Autodesk Inventor part; units mm, degrees
ref_plane "YZ Plane" through (0, 0, 0) normal (1, 0, 0) x (0, 1, 0)
ref_plane "XZ Plane" through (0, 0, 0) normal (0, 1, 0) x (-1, 0, 0)
ref_plane "XY Plane" through (0, 0, 0) normal (0, 0, 1) x (1, 0, 0)
sketch "Boceto1" plane through (0, 0, 0) normal (0, 1, 0) x (-1, 0, 0)
  line L0 (0, 0) -> (22, 0)
  line L1 (22, 0) -> (22, -15)
  line L2 (22, -15) -> (0, -15)
  line L3 (0, -15) -> (-12, -15)
  line L4 (-12, -15) -> (-12, 0)
  line L5 (-12, 0) -> (0, 0)
  dimension "d15" = 12
extrude "Extrusión1" add sketch "Boceto1" along normal blind 3
sketch "Boceto3" plane through (0, 3, 0) normal (0, 1, 0) x (1, 0, 0)
  line L0 (-22, 15) -> (-22, 0)
  line L1 (-22, 15) -> (-27, 15)
  line L2 (-27, 15) -> (-27, 0)
  line L3 (-27, 0) -> (-22, 0)
  line L4 (-22, 0) -> (-22, 15)
  point P0 (0, 0)
  dimension "d4" = 5
extrude "Extrusión2" add sketch "Boceto3" against normal blind 57
sketch "Boceto4" plane through (-22, -54, 0) normal (1, 0, 0) x (0, 0, -1)
  point P0 (0, 54)
sketch "Boceto5" plane through (-22, -54, 0) normal (1, 0, 0) x (0, 0, -1)
  line L0 (0, 57) -> (0, 0)
  line L1 (15, 57) -> (15, 0)
  line L2 (0, 0) -> (15, 0)
  line L3 (15, 0) -> (15, 3.0333)
  line L4 (15, 3.0333) -> (0, 3.0333)
  line L5 (0, 3.0333) -> (0, 0)
  point P0 (0, 54)
extrude "Extrusión3" add sketch "Boceto5" along normal blind 12
sketch "Boceto7" plane through (12, 0, 0) normal (1, 0, 0) x (0, 0, -1)
  line L0 (0, 0) -> (0, -50.9667)
  line L1 (0, 3) -> (0, 0)
  line L2 (0, 0) -> (0, -7)
  line L3 (0, -7) -> (10.8666, -7)
  line L4 (0, -7) -> (0, -13)
  line L5 (0, -13) -> (15, -13)
  line L6 (15, 0) -> (15, -50.9667)
  line L7 (15, 3) -> (15, -54)
  line L8 (15, 3) -> (15, -13)
  line L9 (15, 3) -> (0, 3)
  line L10 (15, 3) -> (0, 3)
  line L11 (0, 3) -> (0, -13)
  line L12 (0, -7) -> (15, -7)
  circle A0 centre (7.5, -7) radius 1.5
  dimension "d16" = 7
  dimension "d17" = 6
  dimension "d18" = 3
extrude "Extrusión5" add sketch "Boceto7" along normal blind 6 contours L1 L9 L7 L6 L12 L3 A0 L0 | L3 A0 L12 L6 L5 L0
sketch "Boceto8" plane through (-22, 0, 0) normal (1, 0, 0) x (0, 0, -1)
  line L0 (15, -50.9667) -> (0, -50.9667)
  line L1 (0, -50.9667) -> (0, -40.9667)
  line L2 (0, 0) -> (0, -50.9667)
  line L3 (0, -40.9667) -> (0, -38.9667)
  line L4 (0, -38.9667) -> (15, -38.9667)
  line L5 (15, 0) -> (15, -50.9667)
  line L6 (0, -40.9667) -> (15, -40.9667)
  line L7 (15, -40.9667) -> (15, -38.9667)
  dimension "d21" = 10
  dimension "d22" = 2
extrude "Extrusión6" add sketch "Boceto8" along normal blind 6 contours L6 L2 L4 L5
sketch "Boceto9" plane through (-22, -38.9667, 0) normal (0, 1, 0) x (1, 0, 0)
  line L0 (0, 0) -> (0, 15)
  line L1 (0, 0) -> (0, 15)
  line L2 (6, 15) -> (6, 0)
  line L3 (0, 15) -> (6, 15)
  line L4 (6, 15) -> (6, 0)
  line L5 (0, 15) -> (0, 0)
  line L6 (6, 0) -> (0, 0)
  point P0 (22, 0)
extrude "Extrusión7" add sketch "Boceto9" along normal blind 18
properties part number "agarre motor"
The model under review builds one solid part; all positions refer to its coordinate system, in mm. A direction names the side the tool comes from. Coordinates: 2 decimals unless noted, no trailing zeros. Loops run counter-clockwise (first coordinate to the right, second up) from the corner with the lowest first, then second, coordinate; pieces in that order, holes last. Notation, with made-up numbers: (4.5, 1) -> (42.5, 1) arc R19 cw to (42.5, 13) -> close; hole circle Ø5 at (21.25, 72.25). An arc over 180 degrees is marked (long way). Use a Markdown table: item, result. Add a question column.
1. Draft analysis for pull direction X (two halves, no side actions). For faces 1 (the face through (-27, -25, -8)), 2 (the face through (-5, 0, -7)), 3 (the face through (-19, -54, -7)), 4 (the face through (-10, -52, -7)), state which applies: pulls with the +X half, pulls with the -X half, needs draft (parallel to the pull), parting line crosses it, or undercut.
2. Add section B-B on y = -7. Write out the cut boundary in (x, z).
3. To check wall thickness, follow line 1 (Y direction, x = -20, z = -4); line 2 (Z direction, x = 15.6, y = -7); line 3 (Y direction, x = 16.2, z = -7.5). State the ranges of each line that lie inside material, in increasing order.
4. Add section A-A on x = -19.5. Write out the cut boundary in (y, z), plus the area to 4 significant figures.
5. Clearance check with flat-ended pins moving along their axes: pin 1 Ø3 at (y, z) = (-44, -6.5) entering from +X; pin 2 Ø1.5 at (y, z) = (-52, -5) entering from +X; pin 3 Ø12 at (x, y) = (5, -3.5) entering from -Z; pin 4 Ø5 at (x, z) = (14.5, -4.5) entering from -Y. State where each tip first meets the part, or that it passes through.
6. Add section D-D on x = 13. Write out the cut boundary in (y, z), plus the area to 3 significant figures.
7. Add section C-C on z = -7.5. Write out the cut boundary in (x, y), plus the area to 3 significant figures.
8. Machinability: for faces 5 (the face through (-19, -20.967, -8)), 6 (the face through (-22, -10, -8)), 7 (the face through (15, -13, -7)), 8 (the face through (15, -6.1, -6.3)), which of the approach directions +Z, -Z, +X, -X, +Y, -Y give a long, thin tool a straight path to every point of the face, cutting with its end or side? Answer none if there is none.
Returned:
| question | item | result |
|---|---|---|
| 1 | face 1 | pulls with the -X half |
| 1 | face 2 | undercut |
| 1 | face 3 | needs draft |
| 1 | face 4 | pulls with the +X half |
| 2 | outline | (-27, -15) -> (-22, -15) -> (-22, 0) -> (-27, 0) -> close; (12, -15) -> (18, -15) -> (18, -9) -> (12, -9) -> close; (12, -6) -> (18, -6) -> (18, 0) -> (12, 0) -> close |
| 3 | line 1 | y = -54 to -50.97, -40.97 to -20.97, 0 to 3 |
| 3 | line 2 | z = -15 to -9, -6 to 0 |
| 3 | line 3 | y = -13 to -8.5, -5.5 to 3 |
| 4 | outline | (-54, -15) -> (-50.97, -15) -> (-50.97, 0) -> (-54, 0) -> close; (-40.97, -15) -> (-20.97, -15) -> (-20.97, 0) -> (-40.97, 0) -> close; (0, -15) -> (3, -15) -> (3, 0) -> (0, 0) -> close |
| 4 | area | 390.5 mm² |
| 5 | pin 1 | stops at x = -22 |
| 5 | pin 2 | stops at x = -10 |
| 5 | pin 3 | stops at z = -15 |
| 5 | pin 4 | stops at y = -13 |
| 6 | outline | (-13, -15) -> (3, -15) -> (3, 0) -> (-13, 0) -> close; hole circle Ø3 at (-7, -7.5) |
| 6 | area | 233 mm² |
| 7 | outline | (-27, -54) -> (-10, -54) -> (-10, -50.97) -> (-22, -50.97) -> (-22, -40.97) -> (-16, -40.97) -> (-16, -20.97) -> (-22, -20.97) -> (-22, 0) -> (12, 0) -> (12, -5.5) -> (18, -5.5) -> (18, 3) -> (-27, 3) -> close; (12, -13) -> (18, -13) -> (18, -8.5) -> (12, -8.5) -> close |
| 7 | area | 621 mm² |
| 8 | face 5 | +Z, -Z, +X |
| 8 | face 6 | +Z, -Z |
| 8 | face 7 | +Z, -Z, +X, -Y |
| 8 | face 8 | +X |
